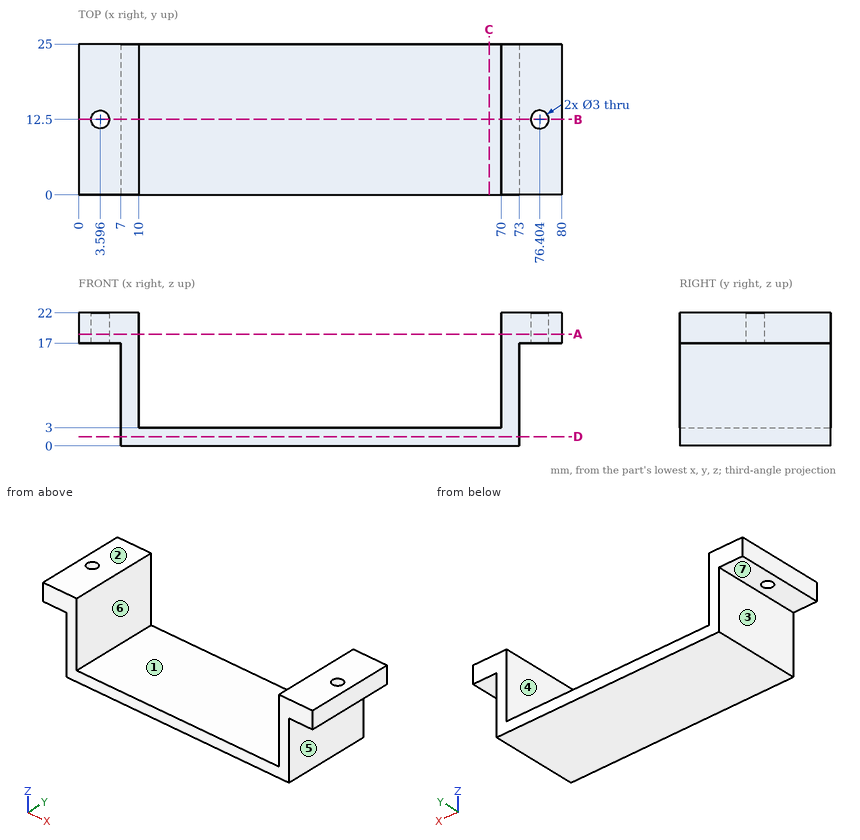
Job drawing, mm, ordinate dimensions from the low corner. One solid piece. A direction names the side the tool comes from. Give positions to 0.01 mm unless a question says otherwise; leave off trailing zeros. Order: outer loops, then holes, each group sorted by start corner. A loop starts at its lowest first (then second) coordinate and runs counter-clockwise, first axis right, second up. Notation, with made-up numbers: (14.5, -10) -> (39.5, -10) arc R14 cw to (39.5, -4) -> close; hole circle Ø9 at (13.5, 27.25). An arc over 180 degrees is marked (long way). Return JSON: item names as keys, results as strings.
Q1. Mould opens along X. For the marked faces 4, 5, 6 and 7 say: pulls with the +X half, pulls with the -X half, needs draft (parallel to the pull), parting line crosses it, or undercut.
Working result:
{"face 4": "undercut", "face 5": "pulls with the +X half", "face 6": "undercut", "face 7": "needs draft"}
Q2. Drill centre lines: line 1 (X direction, y = 9.25, z = 12.25); line 2 (X direction, y = 19, z = 21); line 3 (Z direction, x = 4.5, y = 14). Where is each one in solid material? Low to high.
Working result:
{"line 1": "7 to 10, 70 to 73", "line 2": "0 to 10, 70 to 80", "line 3": "17 to 22"}
Q3. Saw through at D-D (z = 1.5). Write the cut outline in (x, y).
Working result:
{"outline": "(7, 0) -> (73, 0) -> (73, 25) -> (7, 25) -> close"}
Q4. Flat gauge pins, fed straight in: pin 1 (1 mm diameter, centred on y = 18, z = 9.5, fed in from -X); pin 2 (4 mm diameter, centred on x = 3.596, y = 12.5, fed in from -Z); pin 3 (4 mm diameter, centred on x = 13.5, y = 19, fed in from +Z). Where does each tip first touch, or does it go through?
Working result:
{"pin 1": "x = 7", "pin 2": "z = 17", "pin 3": "z = 3"}
Q5. Saw through at B-B (y = 12.5). Write the cut outline in (x, z).
Working result:
{"outline": "(0, 17) -> (2.1, 17) -> (2.1, 22) -> (0, 22) -> close; (5.1, 17) -> (7, 17) -> (7, 0) -> (73, 0) -> (73, 17) -> (74.9, 17) -> (74.9, 22) -> (70, 22) -> (70, 3) -> (10, 3) -> (10, 22) -> (5.1, 22) -> close; (77.9, 17) -> (80, 17) -> (80, 22) -> (77.9, 22) -> close"}
Q6. Which spindle directions (+Z, -Z, +X, -X, +Y, -Y) get a long thin tool onto all of the face, cutting with end or side? Do the marked faces 1, 2 and 3. Say none if no direction does.
Working result:
{"face 1": "+Z, +Y, -Y", "face 2": "+Z, +X, -X, +Y, -Y", "face 3": "-Z, -X, +Y, -Y"}
Q7. Saw through at C-C (x = 68). Write the cut outline in (y, z).
Working result:
{"outline": "(0, 0) -> (25, 0) -> (25, 3) -> (0, 3) -> close"}
Q8. Saw through at A-A (z = 18.5). Write the cut outline in (x, y), then the cut area to 3 significant figures.
Working result:
{"outline": "(0, 0) -> (10, 0) -> (10, 25) -> (0, 25) -> close; (70, 0) -> (80, 0) -> (80, 25) -> (70, 25) -> close; hole circle Ø3 at (3.6, 12.5); hole circle Ø3 at (76.4, 12.5)", "area": "486 mm²"}
